from build123d import *

# Parameters (mm, degrees)
SKETCH_W        = 114
SKETCH_H        = 80
PAD_DEPTH       = 61
SKETCH001_W     = 110
SKETCH001_H     = 57
POCKET_DEPTH    = 78
POCKET001_DEPTH = 2
POCKET002_DEPTH = 90
SKETCH004_W     = 30
SKETCH004_H     = 6
PAD001_DEPTH    = 2
SKETCH005_W     = 30
SKETCH005_H     = 2
PAD002_DEPTH    = 30
FILLET_R        = 1
FILLET001_R     = 1
FILLET002_R     = 1
FILLET003_R     = 1
FILLET004_R     = 1
FILLET005_R     = 0.5
FILLET006_R     = 1
FILLET007_R     = 1
FILLET008_R     = 1
FILLET009_R     = 1
FILLET010_R     = 1


with BuildPart() as part:
    # Sketch → Pad (new body)
    with BuildSketch(Plane.XY):
        with Locations((57, 40)):
            Rectangle(SKETCH_W, SKETCH_H)
    extrude(amount=PAD_DEPTH)

    # Sketch001 (on Face1 of Pad) → Pocket (cut)
    with BuildSketch(Plane(origin=(0, 80, 0), x_dir=(-1, 0, 0), z_dir=(0, 1, 0))):
        with Locations((-57, 30.5)):
            Rectangle(SKETCH001_W, SKETCH001_H)
    extrude(amount=-POCKET_DEPTH, mode=Mode.SUBTRACT)

    # Sketch002 (on Face4 of Pocket) → Pocket001 (cut)
    with BuildSketch(Plane.XY.offset(61)):
        Polygon((32, 80), (43.5, 20), (70.5, 20), (82, 80), align=None)
    extrude(amount=-POCKET001_DEPTH, mode=Mode.SUBTRACT)

    # Sketch003 (on Face4 of Pocket001) → Pocket002 (cut)
    with BuildSketch(Plane.XY.offset(61)):
        Polygon((0, 70), (23.734643, 70), (35.234643, 10), (52, 10), (52, 0), (0, 0), align=None)
        Polygon((78.765357, 10), (90.265357, 70), (114, 70), (114, 0), (62, 0), (62, 10), align=None)
    extrude(amount=-POCKET002_DEPTH, mode=Mode.SUBTRACT)

    # Sketch004 (on Face1 of Pocket002) → Pad001 (join)
    with BuildSketch(Plane(origin=(0, 80, 0), x_dir=(-1, 0, 0), z_dir=(0, 1, 0))):
        with Locations((-57, -3)):
            Rectangle(SKETCH004_W, SKETCH004_H)
    extrude(amount=-PAD001_DEPTH)

    # Sketch005 (on Face23 of Pad001) → Pad002 (join)
    with BuildSketch(Plane.XZ.offset(-78)):
        with Locations((57, -5)):
            Rectangle(SKETCH005_W, SKETCH005_H)
    extrude(amount=PAD002_DEPTH)

    # Fillet
    fillet_edges = [part.edges().sort_by_distance(p)[0] for p in [
        (78.765357, 10, 1),
    ]]
    fillet(fillet_edges, radius=FILLET_R)

    # Fillet001
    fillet001_edges = [part.edges().sort_by_distance(p)[0] for p in [
        (114, 75, 0),
    ]]
    fillet(fillet001_edges, radius=FILLET001_R)

    # Fillet002
    fillet002_edges = [part.edges().sort_by_distance(p)[0] for p in [
        (114, 75, 61),
    ]]
    fillet(fillet002_edges, radius=FILLET002_R)

    # Fillet003
    fillet003_edges = [part.edges().sort_by_distance(p)[0] for p in [
        (57, 80, -6),
    ]]
    fillet(fillet003_edges, radius=FILLET003_R)

    # Fillet004
    fillet004_edges = [part.edges().sort_by_distance(p)[0] for p in [
        (57, 48, -6),
    ]]
    fillet(fillet004_edges, radius=FILLET004_R)

    # Fillet005
    fillet005_edges = [part.edges().sort_by_distance(p)[0] for p in [
        (57, 48, -4),
    ]]
    fillet(fillet005_edges, radius=FILLET005_R)

    # Fillet006
    fillet006_edges = [part.edges().sort_by_distance(p)[0] for p in [
        (0, 75, 0),
    ]]
    fillet(fillet006_edges, radius=FILLET006_R)

    # Fillet007
    fillet007_edges = [part.edges().sort_by_distance(p)[0] for p in [
        (0, 75, 61),
    ]]
    fillet(fillet007_edges, radius=FILLET007_R)

    # Fillet008
    fillet008_edges = [part.edges().sort_by_distance(p)[0] for p in [
        (78.765357, 10, 60),
        (35.234643, 10, 60),
    ]]
    fillet(fillet008_edges, radius=FILLET008_R)

    # Fillet009
    fillet009_edges = [part.edges().sort_by_distance(p)[0] for p in [
        (57, 0, 61),
        (57, 0, 0),
    ]]
    fillet(fillet009_edges, radius=FILLET009_R)

    # Fillet010
    fillet010_edges = [part.edges().sort_by_distance(p)[0] for p in [
        (35.234643, 10, 1),
    ]]
    fillet(fillet010_edges, radius=FILLET010_R)


solid = part.part
CAD build for the part. Positions are in the model's coordinates, mm. A direction names the side the tool comes from. Round coordinates to 2 decimals unless told otherwise and drop trailing zeros. Loops run counter-clockwise (first coordinate to the right, second up) from the corner with the lowest first, then second, coordinate; pieces in that order, holes last. Notation, with made-up numbers: M 81,-28.75 L 113,-28.75 A6 cw 113,-21.75 Z; hole C 12,14 d1. An arc over 180 degrees is marked long. One line per question, with ' | ' between items. Start each with the question number.
Item 1: Cut at A-A, the plane x = 96.5. Write the cut outline in (y, z), plus the area to 3 significant figures.
Item 2: Wall check: line 1 (X direction, y = 71.5, z = 42.5); line 2 (Z direction, x = 56, y = 13); line 3 (Z direction, x = 62, y = 43.5). Give the ranges that are in metal, low to high.
Item 3: Cut at B-B, the plane z = 50. Write the cut outline in (x, y).
Item 4: Cut at C-C, the plane y = 41. Write the cut outline in (x, z) (3 decimals).
Item 5: Two-plate mould, pull along X, no slides. Class faces 4 (the flat face through (57, 64, -6)), 5 (the flat face through (2, 75, 30)), 6 (the flat face through (29.327, 40.82, 60.014)): pulls with the +X half, pulls with the -X half, needs draft (parallel to the pull), parting line crosses it, or undercut.
Item 6: Pin check, flat tips, straight feed: pin 1 Ø2 at (x, z) = (55, -2.5) entering from -Y; pin 2 Ø9 at (x, y) = (60.5, 70.5) entering from +Z; pin 3 Ø0.6 at (x, z) = (71.5, 60) entering from -Y; pin 4 Ø23.5 at (x, y) = (63.5, 41) entering from -Z. Stop position of each tip, or through.
Item 7: Cut at D-D, the plane y = 17. Write the cut outline in (x, z).
Item 8: Which spindle directions (+Z, -Z, +X, -X, +Y, -Y) get a long thin tool onto all of the face, cutting with end or side? Do faces 1 (the flat face through (57, 78, -2)), 2 (the flat face through (1, 70, 31)), 3 (the flat face through (112, 75, 30)). Say none if no direction does.
Responses:
1) outline: M 70,0 L 80,0 L 80,2 L 70,2 Z; M 70,59 L 80,59 L 80,61 L 70,61 Z | area: 40.0 mm²
2) line 1: x = 0 to 2, 112 to 114 | line 2: z = 0 to 2, 59 to 61 | line 3: z = 0 to 2
3) outline: M 0,70 L 2,70 L 2,80 L 0,80 Z; M 52,0 L 62,0 L 62,2 L 52,2 Z; M 112,70 L 114,70 L 114,80 L 112,80 Z
4) outline: M 29.293,0 L 84.707,0 L 84.707,2 L 29.293,2 Z; M 29.293,59 L 39.475,59 L 39.475,61 L 29.293,61 Z; M 74.525,59 L 84.707,59 L 84.707,61 L 74.525,61 Z
5) face 4: needs draft | face 5: undercut | face 6: pulls with the -X half
6) pin 1: stops at y = 78 | pin 2: stops at z = 2 | pin 3: stops at y = 10 | pin 4: stops at z = -6
7) outline: M 33.89,0 L 80.11,0 L 80.11,2 L 33.89,2 Z; M 33.89,59 L 80.11,59 L 80.11,61 L 33.89,61 Z
8) face 1: +X, -X, -Y | face 2: +Z, -Z, -X, -Y | face 3: +Y, -Y
